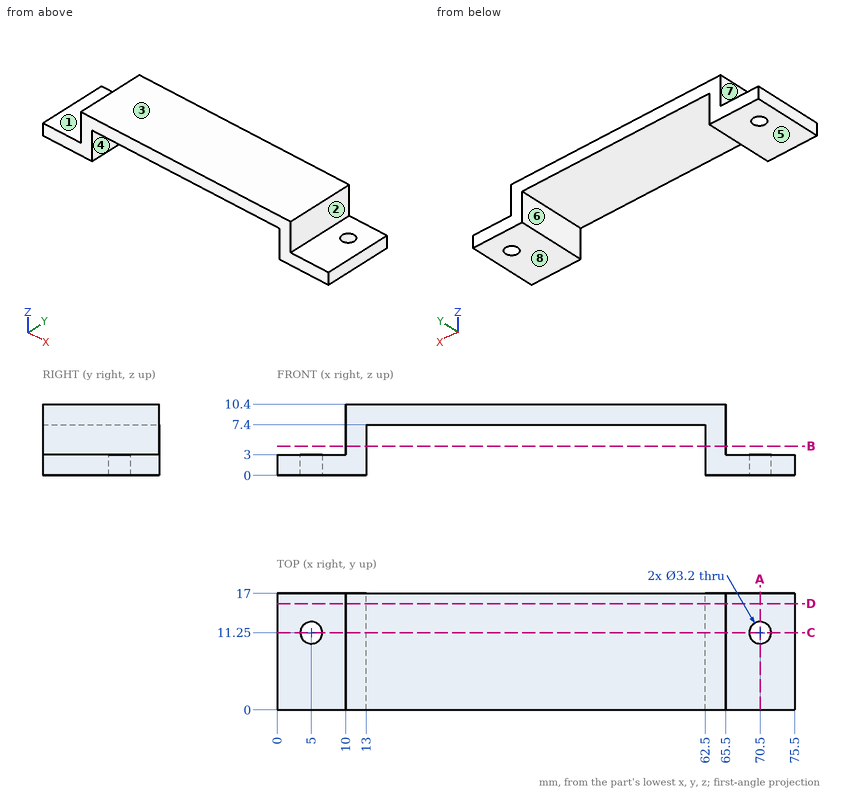
Drawing for the job (mm, zero at the part's lowest x, y, z). A direction names the side the tool comes from. Give positions to 0.01 mm unless a question says otherwise; leave off trailing zeros. Write each loop counter-clockwise with the first axis right and the second up, starting at its lowest first coordinate (ties: lowest second). Pieces come first, ordered by that corner, then holes. Notation, with made-up numbers: M -2.5,70.25 L 22.5,70.25 A20 ccw 22.5,80.25 Z; hole C 34.25,-30.75 d10. An arc over 180 degrees is marked long. Return JSON: item names as keys, results as strings. Group by question number.
(1) Band-saw the part on A-A (x = 70.5). Give the cut face in (y, z), and give its area (3 significant figures).
(2) Band-saw the part on D-D (y = 15.5). Give the cut face in (x, z).
(3) Flat gauge pins, fed straight in: pin 1 Ø2 at (y, z) = (11, 7.5) entering from -X; pin 2 Ø5 at (x, y) = (4, 5.5) entering from +Z; pin 3 Ø10 at (x, y) = (24.5, 2.5) entering from -Z. Where does each tip first touch, or does it go through?
(4) 3-axis set-ups, long thin cutter, end or side, ignore diameter. For the marked faces 1, 2, 3, 4 and 5: which of +Z, -Z, +X, -X, +Y, -Y reach the whole face in a straight line?
(5) Drill centre lines: L1, parallel to X at y = 6.5, z = 1; L2, parallel to X at y = 2.5, z = 5; L3, parallel to Y at x = 5, z = 1.55. Where is each one in solid material? Low to high. Write a range as [from, to].
(6) Band-saw the part on B-B (z = 4.25). Give the cut face in (x, y).
(7) Mould opens along X. For the marked faces 6, 7 and 8 say: pulls with the +X half, pulls with the -X half, needs draft (parallel to the pull), parting line crosses it, or undercut.
(8) Band-saw the part on C-C (y = 11.25). Give the cut face in (x, z).
Entries:
{
 "1": {"outline": "M 0,0 L 9.65,0 L 9.65,3 L 0,3 Z; M 12.85,0 L 17,0 L 17,3 L 12.85,3 Z", "area": "41.4 mm^2"},
 "2": {"outline": "M 0,0 L 13,0 L 13,7.4 L 62.5,7.4 L 62.5,0 L 75.5,0 L 75.5,3 L 65.5,3 L 65.5,10.4 L 10,10.4 L 10,3 L 0,3 Z"},
 "3": {"pin 1": "stops at x = 10", "pin 2": "stops at z = 3", "pin 3": "stops at z = 7.4"},
 "4": {"face 1": "+Z, -X, +Y, -Y", "face 2": "+Z, +X, +Y, -Y", "face 3": "+Z, +X, -X, +Y, -Y", "face 4": "-Z, +Y, -Y", "face 5": "-Z, +X, -X, +Y, -Y"},
 "5": {"L1": "x = [0, 13], [62.5, 75.5]", "L2": "x = [10, 13], [62.5, 65.5]", "L3": "y = [0, 9.65], [12.85, 17]"},
 "6": {"outline": "M 10,0 L 13,0 L 13,17 L 10,17 Z; M 62.5,0 L 65.5,0 L 65.5,17 L 62.5,17 Z"},
 "7": {"face 6": "undercut", "face 7": "pulls with the -X half", "face 8": "needs draft"},
 "8": {"outline": "M 0,0 L 3.4,0 L 3.4,3 L 0,3 Z; M 6.6,0 L 13,0 L 13,7.4 L 62.5,7.4 L 62.5,0 L 68.9,0 L 68.9,3 L 65.5,3 L 65.5,10.4 L 10,10.4 L 10,3 L 6.6,3 Z; M 72.1,0 L 75.5,0 L 75.5,3 L 72.1,3 Z"}
}
